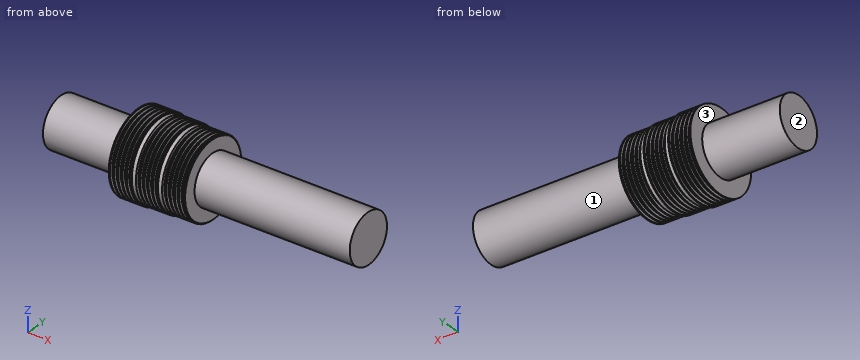
```python
from build123d import *


with BuildPart() as part:
    # Sketch1 → Revolve1 (revolve)
    with BuildSketch(Plane.XY):
        Polygon((19.05, 9.809988), (19.304, 9.809988), (19.304, 9.022588), (20.0914, 9.022588), (20.0914, 9.809988), (20.3454, 9.809988), (20.3454, 9.022588), (21.1328, 9.022588), (21.1328, 9.809988), (21.3868, 9.809988), (21.3868, 9.022588), (22.1742, 9.022588), (22.1742, 9.809988), (22.4282, 9.809988), (22.4282, 9.022588), (23.2156, 9.022588), (23.2156, 9.809988), (23.4696, 9.809988), (23.4696, 9.022588), (24.257, 9.022588), (24.257, 9.809988), (24.511, 9.809988), (24.511, 9.555988), (25.527, 9.555988), (25.527, 8.768588), (26.3144, 8.768588), (26.3144, 9.555988), (26.5684, 9.555988), (26.5684, 8.768588), (27.3558, 8.768588), (27.3558, 9.555988), (27.6098, 9.555988), (27.6098, 8.768588), (28.3972, 8.768588), (28.3972, 9.555988), (28.6512, 9.555988), (28.6512, 8.768588), (29.4386, 8.768588), (29.4386, 9.555988), (29.6926, 9.555988), (29.6926, 8.768588), (30.48, 8.768588), (30.48, 9.555988), (30.734, 9.555988), (30.734, 9.301988), (31.75, 9.301988), (31.75, 8.514588), (32.5374, 8.514588), (32.5374, 9.301988), (32.7914, 9.301988), (32.7914, 8.514588), (33.5788, 8.514588), (33.5788, 9.301988), (33.8328, 9.301988), (33.8328, 8.514588), (34.6202, 8.514588), (34.6202, 9.301988), (34.8742, 9.301988), (34.8742, 8.514588), (35.6616, 8.514588), (35.6616, 9.301988), (35.9156, 9.301988), (35.9156, 8.514588), (36.703, 8.514588), (36.703, 9.301988), (36.957, 9.301988), (36.957, 9.047988), (37.211, 9.047988), (37.211, 5.999988), (75.311, 5.999988), (75.311, 0), (61.976, 0), (0, 0), (0, 5.999988), (19.05, 5.999988), align=None)
    revolve(axis=Axis((0, 0, 0), (1, 0, 0)))


solid = part.part
```
Geometry check sheet. Reference: the model listing, model coordinates, mm. Face numbers are marked on the shaded views. A direction names the side the tool comes from. Round coordinates to 2 decimals unless told otherwise and drop trailing zeros. Loops run counter-clockwise (first coordinate to the right, second up) from the corner with the lowest first, then second, coordinate; pieces in that order, holes last. Notation, with made-up numbers: (35.25, -27.5) - (75.25, -27.5) arc R16 ccw to (75.25, -19.5) - close; hole circle Ø3 at (3, -16.75). An arc over 180 degrees is marked (long way). Write item = value, one per line. Start each with the question number.
1. Set-up check for the marked faces 1, 2 and 3: record each of +Z, -Z, +X, -X, +Y, -Y from which the full face is reachable in a straight line by a thin tool's end or side.
2. Section check A-A on x = 40.5. Enter the section's corners in (y, z), then the cut area to 3 significant figures.
3. Thickness scan on line 1 (X direction, y = -6.25, z = -4.5); line 2 (Y direction, x = 20, z = 7.25); line 3 (Y direction, x = 59, z = -5.5). Record the ranges inside material, lowest first.
4. Depth check by flat-ended pin: pin 1 (4 mm diameter, centred on x = 43, y = 5.5, fed in from -Z); pin 2 (10 mm diameter, centred on x = 49, y = -5, fed in from -Z); pin 3 (1 mm diameter, centred on x = 10, y = -3, fed in from -Z). Enter the tip coordinate at first touch or a pass-through.
Working result:
q1.face_1 = +X
q1.face_2 = +Z, -Z, -X, +Y, -Y
q1.face_3 = -X
q2.outline = circle Ø12 at (0, 0)
q2.area = 113 mm^2
q3.line_1 = 19.05 to 37.21
q3.line_2 = -5.37 to 5.37
q3.line_3 = -2.4 to 2.4
q4.pin_1 = -4.87
q4.pin_2 = -6
q4.pin_3 = -5.45
